```python
from build123d import *

# Parameters (mm, degrees)
SKETCH1_R                = 7.5
SKETCH1_R_2              = 12.5
BOSS_EXTRUDE1_DEPTH      = 10
M5_CLEARANCE_HOLE2_D     = 5.5
M5_CLEARANCE_HOLE2_DEPTH = 30
M5_CLEARANCE_HOLE2_TIP   = 1.652366702
M8_CLEARANCE_HOLE1_D     = 9
M8_CLEARANCE_HOLE1_DEPTH = 30
M8_CLEARANCE_HOLE1_TIP   = 2.703872786
M6_CLEARANCE_HOLE1_D     = 6.6
M6_CLEARANCE_HOLE1_DEPTH = 30
M6_CLEARANCE_HOLE1_TIP   = 1.982840043


with BuildPart() as part:
    # Sketch1 → Boss-Extrude1 (new body)
    with BuildSketch(Plane(origin=(0, 0, 0), x_dir=(0, 0, -1), z_dir=(1, 0, 0))):
        with BuildLine():
            Line((10, 215.979685497), (10, 250))
            Line((10, 250), (25, 250))
            Line((25, 250), (35, 250))
            Line((35, 250), (35, 208.897946033))
            Line((35, 208.897946033), (25.122964317, 208.897946033))
            ThreePointArc((25.122964317, 208.897946033), (13.508598299, 107.244900729), (24.385178415, 5.510269837))
            ThreePointArc((24.385178415, 5.510269837), (6.422608809, -24.160920845), (-23.902542108, -7.325877476))
            add(Edge.make_bspline(
                [(-23.902542108, -7.325877476), (-48.990185726, 110.151133061), (10, 215.979685497)],
                knots=[0, 0, 0, 1, 1, 1], degree=2))
        make_face()
        with Locations((5, 180)):
            Circle(SKETCH1_R, mode=Mode.SUBTRACT)
        with Locations((-2.5, 140)):
            Circle(SKETCH1_R_2, mode=Mode.SUBTRACT)
        with BuildLine():
            Line((-24.338949666, 59.866716225), (-19.390233073, 94.152430511))
            ThreePointArc((-19.390233073, 94.152430511), (-7.01844159, 104.866716225), (5.353349892, 94.152430511))
            Line((5.353349892, 94.152430511), (10.302066485, 59.866716225))
            ThreePointArc((10.302066485, 59.866716225), (-7.01844159, 39.866716225), (-24.338949666, 59.866716225))
        make_face(mode=Mode.SUBTRACT)
    extrude(amount=BOSS_EXTRUDE1_DEPTH)

    # M5 Clearance Hole2
    with Locations(Plane(origin=(0, 0, -35), x_dir=(-1, 0, 0), z_dir=(0, 0, -1))):
        with Locations((-4.98385201, 238), (-4.98385201, 222)):
            Hole(M5_CLEARANCE_HOLE2_D / 2, depth=M5_CLEARANCE_HOLE2_DEPTH)
            with Locations((0, 0, -(M5_CLEARANCE_HOLE2_DEPTH + M5_CLEARANCE_HOLE2_TIP / 2))):  # 118° drill point
                Cone(0, M5_CLEARANCE_HOLE2_D / 2, M5_CLEARANCE_HOLE2_TIP, mode=Mode.SUBTRACT)

    # M8 Clearance Hole1
    with Locations(Plane(origin=(10, 0, 0), x_dir=(0, 0, -1), z_dir=(1, 0, 0))):
        with Locations((0, 0)):
            Hole(M8_CLEARANCE_HOLE1_D / 2, depth=M8_CLEARANCE_HOLE1_DEPTH)
            with Locations((0, 0, -(M8_CLEARANCE_HOLE1_DEPTH + M8_CLEARANCE_HOLE1_TIP / 2))):  # 118° drill point
                Cone(0, M8_CLEARANCE_HOLE1_D / 2, M8_CLEARANCE_HOLE1_TIP, mode=Mode.SUBTRACT)

    # M6 Clearance Hole1
    with Locations(Plane.ZY):
        with Locations((15, 25)):
            Hole(M6_CLEARANCE_HOLE1_D / 2, depth=M6_CLEARANCE_HOLE1_DEPTH)
            with Locations((0, 0, -(M6_CLEARANCE_HOLE1_DEPTH + M6_CLEARANCE_HOLE1_TIP / 2))):  # 118° drill point
                Cone(0, M6_CLEARANCE_HOLE1_D / 2, M6_CLEARANCE_HOLE1_TIP, mode=Mode.SUBTRACT)


solid = part.part
```
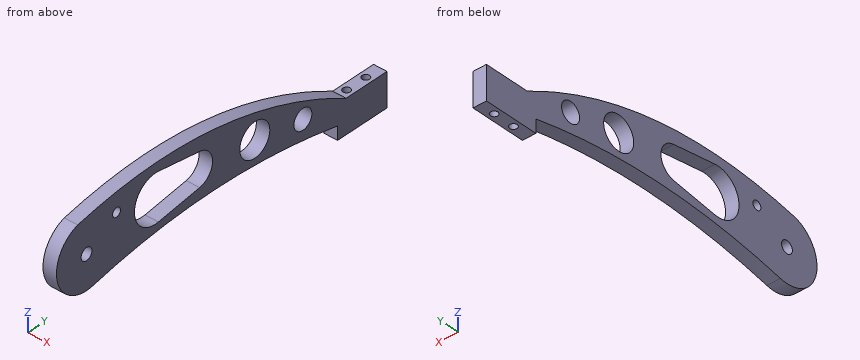
CAD build for the part. Positions are in the model's coordinates, mm. Round coordinates to 2 decimals unless told otherwise and drop trailing zeros. Write each loop counter-clockwise with the first axis right and the second up, starting at its lowest first coordinate (ties: lowest second). Pieces come first, ordered by that corner, then holes. Notation, with made-up numbers: (-26.75, 19.25) - (-13.75, 19.25) arc R28 cw to (-13.75, 51.25) - close; hole circle Ø11 at (89, -34.5). An arc over 180 degrees is marked (long way). Return JSON: item names as keys, results as strings. Group by question number.
Item 1: Band-saw the part on B-B on x = 5. State how many separate pieces and enclosed holes the cut face has, plus the area to 3 significant figures.
Item 2: Probe probe 1 along X at (y, z) = (222, -25.5); probe 2 along Y at (x, z) = (4, 0); probe 3 along Z at (x, y) = (9.75, 175.5). List the from-to ranges inside material, lowest first.
Item 3: Band-saw the part on A-A on y = 238. List the corners of the cut face in (x, z), plus the area to 4 significant figures.
Item 4: Flat gauge pins, fed straight in: pin 1 Ø5 at (x, y) = (9, 166) entering from -Z; pin 2 Ø3 at (x, y) = (5.5, 68) entering from -Z. Where does each tip first touch, or does it go through?
Resolved:
{
 "1": {"separate pieces": "3", "enclosed holes": "5", "area": "7,460 mm²"},
 "2": {"probe 1": "x = 0 to 2.23, 7.73 to 10", "probe 2": "y = -25 to -4.5, 4.5 to 41.34, 102.71 to 127.75, 152.25 to 174.41, 185.59 to 196.71", "probe 3": "z = -18.79 to -11, 1 to 9.32"},
 "3": {"outline": "(0, -35) - (2.23, -35) - (2.23, -10) - (0, -10) - close; (7.73, -35) - (10, -35) - (10, -10) - (7.73, -10) - close", "area": "112.5 mm²"},
 "4": {"pin 1": "stops at z = -17.78", "pin 2": "stops at z = -15.15"}
}
